Drawing for the job (mm, zero at the part's lowest x, y, z). A direction names the side the tool comes from. Round coordinates to 2 decimals unless told otherwise and drop trailing zeros. Write each loop counter-clockwise with the first axis right and the second up, starting at its lowest first coordinate (ties: lowest second). Pieces come first, ordered by that corner, then holes. Notation, with made-up numbers: M 14.5,72 L 46.5,72 A13 cw 46.5,96 Z; hole C -4.75,20.5 d4. An arc over 180 degrees is marked long. Use a Markdown table: item, result. Add a question column.
1) Wall check: probe 1 along X at (y, z) = (9, 25); probe 2 along Z at (x, y) = (28, 18.5). Give the ranges that are in metal, low to high.
2) Two-plate mould, pull along Y, no slides. Class the marked faces 1, 2 and 3: released by +Y, released by -Y, zero draft, split by the parting line, or undercut.
3) Slice it at B-B on z = 22.5. Write the cut outline in (x, y), plus the area to 3 significant figures.
4) Slice it at D-D on y = 44. Write the cut outline in (x, z).
5) Which spindle directions (+Z, -Z, +X, -X, +Y, -Y) get a long thin tool onto all of the face, cutting with end or side? Do the marked faces 4, 5, 6, 7 and 8. Say none if no direction does.
6) Drop flat-ended pins along their axis: P1, Ø8.5, axis at x = 33, z = 61.5, coming from the -Y side; P2, Ø14, axis at x = 18, z = 60, coming from the +Y side; P3, Ø12, axis at x = 20, y = 31, coming from the -Z side; P4, Ø1.5, axis at y = 44, z = 67, coming from the -X side (3 decimals). Give the stop position or say it passes through.
7) Slice it at A-A on y = 20.5. Write the cut outline in (x, z).
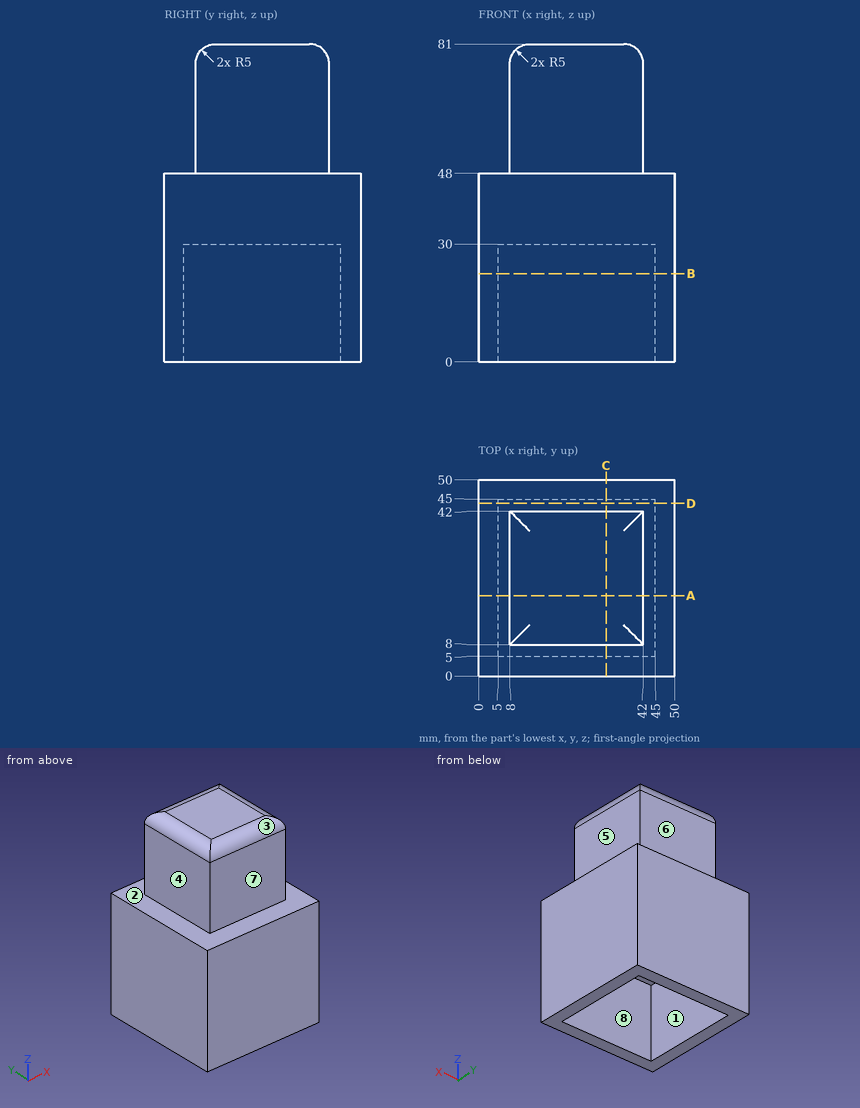
Entries:
| question | item | result |
|---|---|---|
| 1 | probe 1 | x = 0 to 5, 45 to 50 |
| 1 | probe 2 | z = 30 to 81 |
| 2 | face 1 | undercut |
| 2 | face 2 | zero draft |
| 2 | face 3 | released by -Y |
| 3 | outline | M 0,0 L 50,0 L 50,50 L 0,50 Z; hole M 5,5 L 45,5 L 45,45 L 5,45 Z |
| 3 | area | 900 mm^2 |
| 4 | outline | M 0,0 L 5,0 L 5,30 L 45,30 L 45,0 L 50,0 L 50,48 L 0,48 Z |
| 5 | face 4 | +Z, -X, +Y, -Y |
| 5 | face 5 | +Z, +X, +Y, -Y |
| 5 | face 6 | +Z, +X, -X, +Y |
| 5 | face 7 | +Z, +X, -X, -Y |
| 5 | face 8 | -Z |
| 6 | P1 | stops at y = 8 |
| 6 | P2 | stops at y = 42 |
| 6 | P3 | stops at z = 30 |
| 6 | P4 | passes through |
| 7 | outline | M 0,0 L 5,0 L 5,30 L 45,30 L 45,0 L 50,0 L 50,48 L 42,48 L 42,76 A5 ccw 37,81 L 13,81 A5 ccw 8,76 L 8,48 L 0,48 Z |
